Autodesk Inventor part; units mm, degrees
ref_plane "YZ Plane" through (0, 0, 0) normal (1, 0, 0) x (0, 1, 0)
ref_plane "XZ Plane" through (0, 0, 0) normal (0, 1, 0) x (-1, 0, 0)
ref_plane "XY Plane" through (0, 0, 0) normal (0, 0, 1) x (1, 0, 0)
sketch "Sketch1" plane through (0, 0, 0) normal (0, 0, 1) x (1, 0, 0)
  circle A0 centre (0, 0) radius 92.5
  dimension "d22" = 185
extrude "Plate1" add sketch "Sketch1" along normal blind 3
sketch "Sketch5" plane through (0, 0, 3) normal (0, 0, 1) x (1, 0, 0)
  circle A0 centre (0, 0) radius 92.5
  circle A1 centre (0, 72.5) radius 9
  circle A2 centre (0, 0) radius 72.5 construction
  dimension "d23" = 18
  dimension "d30" = 20
extrude "Cut1" cut sketch "Sketch5" against normal blind 3 contours A1
pattern_circular "Circular Pattern1" count 8 over 360 about axis through (0, 0, 0) along (0, 0, 1) of "Cut1"
sketch "Sketch6" plane through (0, 0, 0) normal (0, 0, -1) x (-1, 0, 0)
  circle A0 centre (0, 0) radius 27.5
  dimension "d31" = 55
extrude "Cut2" cut sketch "Sketch6" against normal blind 3
equation "\"d25\" = Thickness"
equation "\"d32\" = Thickness"
equation "\"d2\" = Thickness"
equation "\"BendReliefWidth\" = Thickness"
equation "\"BendReliefDepth\" = 0.5 * Thickness"
equation "\"CornerReliefSize\" = 4 * Thickness"
equation "\"MinimumRemnant\" = 2 * Thickness"
equation "\"TransitionRadius\" = BendRadius"
equation "\"JacobiRadiusSize\" = BendRadius"
equation "\"GapSize\" = Thickness"
properties part number "MSC 922 plug 76 hole" material "Stainless Steel"
Input: part model. Units: mm. Frame: model coordinates. Round coordinates to 2 decimals unless told otherwise and drop trailing zeros. Loops run counter-clockwise (first coordinate to the right, second up) from the corner with the lowest first, then second, coordinate; pieces in that order, holes last. Notation, with made-up numbers: (84, 58) - (126, 58) arc R19 cw to (126, 72) - close; hole circle Ø1 at (78.25, 18). An arc over 180 degrees is marked (long way). One line per item, written item: value. Start each with the question number.
(1) Ray query, line 1 (Y direction, x = 0, z = 1.75); line 2 (X direction, y = 52.5, z = 0.35); line 3 (X direction, y = 2.5, z = 1.85). Return the intervals inside material, ascending. Write a range as [from, to].
(2) Section B-B, the plane y = 75. Return loops of the section in (x, z).
(3) Section C-C, the plane x = 1.5. Return loops of the section in (y, z), plus the area to 3 significant figures.
(4) Section A-A, the plane y = 0. Return loops of the section in (x, z), plus the area to 3 significant figures.
(5) Draft query along Y for faces 1 (the flat face through (-22, -19, 3)), 2 (the cylindrical face through (49.727, -77.996, 1.479)), 3 (the cylindrical face through (-63.714, -1.951, 1.521)). Return one class per face: +Y half, -Y half, draft (parallel to the pull), parting line (faces both ways), or undercut.
(6) Section D-D, the plane z = 0.7. Count the separate pieces of the cut face and the enclosed holes in it, plus the area to 3 significant figures.
Results below:
1. line 1: [-92.5, -81.5], [-63.5, -27.5], [27.5, 63.5], [81.5, 92.5]
1. line 2: [-76.16, -60.18], [-42.35, 42.35], [60.18, 76.16]
1. line 3: [-92.47, -81.15], [-63.85, -27.39], [27.39, 63.85], [81.15, 92.47]
2. outline: (-54.14, 0) - (-8.65, 0) - (-8.65, 3) - (-54.14, 3) - close; (8.65, 0) - (54.14, 0) - (54.14, 3) - (8.65, 3) - close
3. outline: (-92.49, 0) - (-81.37, 0) - (-81.37, 3) - (-92.49, 3) - close; (-63.63, 0) - (-27.46, 0) - (-27.46, 3) - (-63.63, 3) - close; (27.46, 0) - (63.63, 0) - (63.63, 3) - (27.46, 3) - close; (81.37, 0) - (92.49, 0) - (92.49, 3) - (81.37, 3) - close
3. area: 284 mm^2
4. outline: (-92.5, 0) - (-81.5, 0) - (-81.5, 3) - (-92.5, 3) - close; (-63.5, 0) - (-27.5, 0) - (-27.5, 3) - (-63.5, 3) - close; (27.5, 0) - (63.5, 0) - (63.5, 3) - (27.5, 3) - close; (81.5, 0) - (92.5, 0) - (92.5, 3) - (81.5, 3) - close
4. area: 282 mm^2
5. face 1: draft
5. face 2: parting line
5. face 3: undercut
6. separate pieces: 1
6. enclosed holes: 9
6. area: 22,500 mm^2
